from build123d import *

# Parameters (mm, degrees)
F1_DEPTH      = 125
F1_DEPTH_BACK = 125
F6_DEPTH      = 5.001
F7_DEPTH      = 5.001
F8_DEPTH      = 2
F9_DEPTH      = 2
F10_DEPTH     = 2
F11_DEPTH     = 2
F12_T1_DEPTH  = 80
F12_T3_DEPTH  = 80
F12_T5_DEPTH  = 105


# Not quite as in the source:
# - a fillet or chamfer that OpenCascade refuses, or shapes differently, is made with other operations: its cross-section is extruded or revolved along the edge and cut away or added


with BuildPart() as f1:
    # F0 (on Front) → F1 (new body, two sides)
    with BuildSketch(Plane.XZ) as f1_sk:
        Polygon((15, -15), (15, 15), (-15, 15), (-15, -15), (-10, -15), (-10, 10), (10, 10), (10, -15), align=None)
    extrude(amount=F1_DEPTH)
    extrude(f1_sk.sketch, amount=-F1_DEPTH_BACK)

    # F2 (on face) → F6 (cut, through all)
    with BuildSketch(Plane(origin=(10, 0, 0), x_dir=(0, -1, 0), z_dir=(-1, 0, 0))):
        with BuildLine():
            Line((-110, -5), (110, -5))
            ThreePointArc((110, -5), (115, 0), (110, 5))
            Line((110, 5), (-110, 5))
            ThreePointArc((-110, 5), (-115, 0), (-110, -5))
        make_face()
    extrude(amount=-F6_DEPTH, mode=Mode.SUBTRACT)

    # F4 (on face) → F7 (cut, through all)
    with BuildSketch(Plane.YZ.offset(-10)):
        with BuildLine():
            Line((110, 5), (-110, 5))
            ThreePointArc((-110, 5), (-115, 0), (-110, -5))
            Line((-110, -5), (110, -5))
            ThreePointArc((110, -5), (115, 0), (110, 5))
        make_face()
    extrude(amount=-F7_DEPTH, mode=Mode.SUBTRACT)

    # F2 (on face) → F8 (cut)
    with BuildSketch(Plane(origin=(10, 0, 0), x_dir=(0, -1, 0), z_dir=(-1, 0, 0))):
        with BuildLine():
            Line((-110, -10), (110, -10))
            ThreePointArc((110, -10), (120, 0), (110, 10))
            Line((110, 10), (-110, 10))
            ThreePointArc((-110, 10), (-120, 0), (-110, -10))
        make_face()
        with BuildLine():
            ThreePointArc((110, 5), (115, 0), (110, -5))
            Line((110, -5), (-110, -5))
            ThreePointArc((-110, -5), (-115, 0), (-110, 5))
            Line((-110, 5), (110, 5))
        make_face(mode=Mode.SUBTRACT)
    extrude(amount=-F8_DEPTH, mode=Mode.SUBTRACT)

    # F3 (on face) → F9 (cut)
    with BuildSketch(Plane.YZ.offset(15)):
        with BuildLine():
            ThreePointArc((-110, 10), (-120, 0), (-110, -10))
            Line((-110, -10), (110, -10))
            ThreePointArc((110, -10), (120, 0), (110, 10))
            Line((110, 10), (-110, 10))
        make_face()
        with BuildLine():
            ThreePointArc((-110, -5), (-115, 0), (-110, 5))
            Line((-110, 5), (110, 5))
            ThreePointArc((110, 5), (115, 0), (110, -5))
            Line((110, -5), (-110, -5))
        make_face(mode=Mode.SUBTRACT)
    extrude(amount=-F9_DEPTH, mode=Mode.SUBTRACT)

    # F5 (on face) → F10 (cut)
    with BuildSketch(Plane(origin=(-15, 0, 0), x_dir=(0, -1, 0), z_dir=(-1, 0, 0))):
        with BuildLine():
            Line((110, 10), (-110, 10))
            ThreePointArc((-110, 10), (-120, 0), (-110, -10))
            Line((-110, -10), (110, -10))
            ThreePointArc((110, -10), (120, 0), (110, 10))
        make_face()
        with BuildLine():
            ThreePointArc((-110, -5), (-115, 0), (-110, 5))
            Line((-110, 5), (110, 5))
            ThreePointArc((110, 5), (115, 0), (110, -5))
            Line((110, -5), (-110, -5))
        make_face(mode=Mode.SUBTRACT)
    extrude(amount=-F10_DEPTH, mode=Mode.SUBTRACT)

    # F4 (on face) → F11 (cut)
    with BuildSketch(Plane.YZ.offset(-10)):
        with BuildLine():
            Line((110, 10), (-110, 10))
            ThreePointArc((-110, 10), (-120, 0), (-110, -10))
            Line((-110, -10), (110, -10))
            ThreePointArc((110, -10), (120, 0), (110, 10))
        make_face()
        with BuildLine():
            ThreePointArc((-110, -5), (-115, 0), (-110, 5))
            Line((-110, 5), (110, 5))
            ThreePointArc((110, 5), (115, 0), (110, -5))
            Line((110, -5), (-110, -5))
        make_face(mode=Mode.SUBTRACT)
    extrude(amount=-F11_DEPTH, mode=Mode.SUBTRACT)

    # F12: fillet of radius 15 on 6 edges, made by hand

    # F12_s2 → F12_t1 (cut)
    with BuildSketch(Plane.YZ.offset(-52.5)):
        with BuildLine():
            ThreePointArc((125, 0), (120.6066017178, -10.6066017178), (110, -15))
            Line((110, -15), (125, -15))
            Line((125, -15), (125, 0))
        make_face()
        with BuildLine():
            ThreePointArc((-125, 0), (-120.6066017178, -10.6066017178), (-110, -15))
            Line((-110, -15), (-125, -15))
            Line((-125, -15), (-125, 0))
        make_face()
    extrude(amount=F12_T1_DEPTH, mode=Mode.SUBTRACT)

    # F12_s4 → F12_t3 (cut)
    with BuildSketch(Plane.YZ.offset(-27.5)):
        with BuildLine():
            ThreePointArc((110, -15), (120.6066017178, -10.6066017178), (125, 0))
            Line((125, 0), (125, -15))
            Line((125, -15), (110, -15))
        make_face()
        with BuildLine():
            ThreePointArc((-110, -15), (-120.6066017178, -10.6066017178), (-125, 0))
            Line((-125, 0), (-125, -15))
            Line((-125, -15), (-110, -15))
        make_face()
    extrude(amount=F12_T3_DEPTH, mode=Mode.SUBTRACT)

    # F12_s6 → F12_t5 (cut)
    with BuildSketch(Plane.YZ.offset(-52.5)):
        with BuildLine():
            ThreePointArc((125, 0), (120.6066017178, 10.6066017178), (110, 15))
            Line((110, 15), (125, 15))
            Line((125, 15), (125, 0))
        make_face()
        with BuildLine():
            ThreePointArc((-125, 0), (-120.6066017178, 10.6066017178), (-110, 15))
            Line((-110, 15), (-125, 15))
            Line((-125, 15), (-125, 0))
        make_face()
    extrude(amount=F12_T5_DEPTH, mode=Mode.SUBTRACT)


solid = f1.part
The model under review builds one solid part; all positions refer to its coordinate system, in mm. A direction names the side the tool comes from. Coordinates: 2 decimals unless noted, no trailing zeros. Write each loop counter-clockwise with the first axis right and the second up, starting at its lowest first coordinate (ties: lowest second). Pieces come first, ordered by that corner, then holes. Notation, with made-up numbers: (12.5, 63.5) - (24.5, 63.5) arc R29 ccw to (24.5, 85.5) - close; hole circle Ø11 at (-33.5, -19.5). An arc over 180 degrees is marked (long way). Answer as a JSON object with one key per item and string values. Group by question number.
1. Add section C-C (x = 6.25). Give the boundary of the cut face in (y, z).
2. Mouldability with a two-part tool opening along X and no side actions: class faces 1 (the face through (0, -2, 15)), 2 (the face through (-12, -2, 7)), 3 (the face through (13, -2, 7)) as pulls with the +X half, pulls with the -X half, needs draft (parallel to the pull), parting line crosses it, or undercut.
3. Clearance check with flat-ended pins moving along their axes: pin 1 Ø1 at (y, z) = (-92.5, -8.5) entering from -X; pin 2 Ø3 at (y, z) = (-6.5, -5.5) entering from +X; pin 3 Ø4 at (x, y) = (-1.5, -22) entering from -Z; pin 4 Ø4 at (y, z) = (92.5, 2.5) entering from -X. State where each tip first meets the part, or that it passes through.
4. Machinability: for faces 4 (the face through (12.5, 115, 0.1)), 5 (the face through (-11, 120, 0)), 6 (the face through (-13, 2, 7)), which of the approach directions +Z, -Z, +X, -X, +Y, -Y give a long, thin tool a straight path to every point of the face, cutting with its end or side? Answer none if there is none.
5. Add section A-A (y = -77). Give the boundary of the cut face in (x, z), plus the area to 3 significant figures.
6. To check wall thickness, follow probe 1 along X at (y, z) = (14, 8.25); probe 2 along X at (y, z) = (92, -13.5). State the ranges of each line that lie inside material, in increasing order.
7. Add section B-B (z = 0). Give the number of separate pieces and of enclosed holes in the cut face, plus the area to 3 significant figures.
Findings:
{
 "1": {"outline": "(-121.18, 10) - (121.18, 10) arc R15 ccw to (110, 15) - (-110, 15) arc R15 ccw to start"},
 "2": {"face 1": "needs draft", "face 2": "undercut", "face 3": "pulls with the +X half"},
 "3": {"pin 1": "x = -13", "pin 2": "x = 13", "pin 3": "z = 10", "pin 4": "through"},
 "4": {"face 4": "+X, -X", "face 5": "none", "face 6": "-X"},
 "5": {"outline": "(-15, -15) - (-10, -15) - (-10, -10) - (-12, -10) - (-12, -5) - (-13, -5) - (-13, -10) - (-15, -10) - close; (-15, 10) - (-13, 10) - (-13, 5) - (-12, 5) - (-12, 10) - (12, 10) - (12, 5) - (13, 5) - (13, 10) - (15, 10) - (15, 15) - (-15, 15) - close; (10, -15) - (15, -15) - (15, -10) - (13, -10) - (13, -5) - (12, -5) - (12, -10) - (10, -10) - close", "area": "220 mm²"},
 "6": {"probe 1": "-13 to -12, 12 to 13", "probe 2": "-15 to -10, 10 to 15"},
 "7": {"separate pieces": "4", "enclosed holes": "0", "area": "120 mm²"}
}
